from build123d import *

# Parameters (mm, degrees)
F0_W      = 80
F0_H      = 70
F1_DEPTH  = 2
F2_W      = 80
F2_H      = 140
F3_DEPTH  = 2
F4_W      = 140
F4_H      = 68
F5_DEPTH  = 2
F6_W      = 140
F6_H      = 68
F7_DEPTH  = 2
F8_R      = 2
F9_DEPTH  = 2
F10_R     = 2
F11_R     = 1.5
F12_DEPTH = 4
F13_DEPTH = 8
F14_DEPTH = 8
F15_W     = 2
F15_H     = 68
F16_DEPTH = 3
F17_W     = 2
F17_H     = 68
F18_DEPTH = 3


with BuildPart() as f1:
    # F0 (on Front) → F1 (new body)
    with BuildSketch(Plane.XZ):
        with Locations((0, 35)):
            Rectangle(F0_W, F0_H)
    extrude(amount=F1_DEPTH)

    # F2 (on Top) → F3 (join)
    with BuildSketch(Plane.XY):
        with Locations((0, 70)):
            Rectangle(F2_W, F2_H)
    extrude(amount=F3_DEPTH)

    # F4 (on face) → F5 (join)
    with BuildSketch(Plane(origin=(-40, 0, 0), x_dir=(0, -1, 0), z_dir=(-1, 0, 0))):
        with Locations((-70, 36)):
            Rectangle(F4_W, F4_H)
    extrude(amount=-F5_DEPTH)

    # F6 (on face) → F7 (join)
    with BuildSketch(Plane.YZ.offset(40)):
        with Locations((70, 36)):
            Rectangle(F6_W, F6_H)
    extrude(amount=-F7_DEPTH)

    # F8 (on face) → F9 (cut)
    with BuildSketch(Plane.XZ.offset(2)):
        with BuildLine():
            Line((-9.5176118745, 43.1033983122), (-15.8934493297, 49.4792357673))
            ThreePointArc((-15.8934493297, 49.4792357673), (-21.4980117445, 34.7076115032), (-15.4937871876, 20.0938751318))
            Line((-15.4937871876, 20.0938751318), (-9.2937080159, 26.640754142))
            ThreePointArc((-9.2937080159, 26.640754142), (-12.4988440375, 34.8300066879), (-9.5176118745, 43.1033983122))
        make_face()
        with BuildLine():
            Line((-16.6012881064, 50.1870745441), (-21.2010083131, 54.7867947507))
            ThreePointArc((-21.2010083131, 54.7867947507), (-28.997318167, 34.6056155159), (-20.6550363783, 14.6439327912))
            Line((-20.6550363783, 14.6439327912), (-16.1821134643, 19.3670475013))
            ThreePointArc((-16.1821134643, 19.3670475013), (-22.4979192675, 34.6940120382), (-16.6012881064, 50.1870745441))
        make_face()
        with Locations((-26, 61)):
            Circle(F8_R)
        with BuildLine():
            ThreePointArc((19.2028843822, 56.731296128), (-0.3943844841, 63.997318167), (-19.7867947507, 56.2010083131))
            Line((-19.7867947507, 56.2010083131), (-15.1870745441, 51.6012881064))
            ThreePointArc((-15.1870745441, 51.6012881064), (-0.3059879618, 57.4979192675), (14.7299614682, 52.0081814179))
            Line((14.7299614682, 52.0081814179), (19.2028843822, 56.731296128))
        make_face()
        with BuildLine():
            ThreePointArc((14.0416351915, 51.2813537874), (-0.2923884968, 56.4980117445), (-14.4792357673, 50.8934493297))
            Line((-14.4792357673, 50.8934493297), (-8.1033983122, 44.5176118745))
            ThreePointArc((-8.1033983122, 44.5176118745), (-0.1699933121, 47.4988440375), (7.8415560198, 44.7344747772))
            Line((7.8415560198, 44.7344747772), (14.0416351915, 51.2813537874))
        make_face()
        with BuildLine():
            Line((9.5176118745, 26.8966016878), (15.8934493297, 20.5207642327))
            ThreePointArc((15.8934493297, 20.5207642327), (21.5, 35), (15.8934493297, 49.4792357673))
            Line((15.8934493297, 49.4792357673), (9.5176118745, 43.1033983122))
            ThreePointArc((9.5176118745, 43.1033983122), (12.5, 35), (9.5176118745, 26.8966016878))
        make_face()
        with BuildLine():
            Line((21.2010083131, 54.7867947507), (16.6012881064, 50.1870745441))
            ThreePointArc((16.6012881064, 50.1870745441), (22.5, 35), (16.6012881064, 19.8129254559))
            Line((16.6012881064, 19.8129254559), (21.2010083131, 15.2132052493))
            ThreePointArc((21.2010083131, 15.2132052493), (29, 35), (21.2010083131, 54.7867947507))
        make_face()
        with Locations((26, 61)):
            Circle(F8_R)
        with Locations((26, 9)):
            Circle(F8_R)
        with BuildLine():
            Line((-15.1870745441, 18.3987118936), (-19.7867947507, 13.7989916869))
            ThreePointArc((-19.7867947507, 13.7989916869), (0, 6), (19.7867947507, 13.7989916869))
            Line((19.7867947507, 13.7989916869), (15.1870745441, 18.3987118936))
            ThreePointArc((15.1870745441, 18.3987118936), (0, 12.5), (-15.1870745441, 18.3987118936))
        make_face()
        with BuildLine():
            ThreePointArc((8.1033983122, 25.4823881255), (0, 22.5), (-8.1033983122, 25.4823881255))
            Line((-8.1033983122, 25.4823881255), (-14.4792357673, 19.1065506703))
            ThreePointArc((-14.4792357673, 19.1065506703), (0, 13.5), (14.4792357673, 19.1065506703))
            Line((14.4792357673, 19.1065506703), (8.1033983122, 25.4823881255))
        make_face()
        with Locations((-26, 9)):
            Circle(F8_R)
    extrude(amount=-F9_DEPTH, mode=Mode.SUBTRACT)

    # F10
    f10_edges = [f1.edges().sort_by_distance(p)[0] for p in [
        (40, 69, 0),
        (-40, 69, 0),
    ]]
    fillet(f10_edges, radius=F10_R)

    # F11 (on face) → F12 (join)
    with BuildSketch(Plane.XY.offset(2)):
        with BuildLine():
            ThreePointArc((-21.15, 117.6), (-23.2839745962, 120.4722813233), (-26.65, 119.2583123952))
            Line((-26.65, 119.2583123952), (-26.65, 115.9416876048))
            ThreePointArc((-26.65, 115.9416876048), (-23.2839745962, 114.7277186767), (-21.15, 117.6))
        make_face()
        with Locations((-24.15, 117.6)):
            Circle(F11_R, mode=Mode.SUBTRACT)
        with BuildLine():
            Line((26.65, 114.6416876048), (26.65, 117.9583123952))
            ThreePointArc((26.65, 117.9583123952), (21.15, 116.3), (26.65, 114.6416876048))
        make_face()
        with Locations((24.15, 116.3)):
            Circle(F11_R, mode=Mode.SUBTRACT)
        with BuildLine():
            ThreePointArc((-21.15, 35), (-23.2839745962, 37.8722813233), (-26.65, 36.6583123952))
            Line((-26.65, 36.6583123952), (-26.65, 33.3416876048))
            ThreePointArc((-26.65, 33.3416876048), (-23.2839745962, 32.1277186767), (-21.15, 35))
        make_face()
        with Locations((-24.15, 35)):
            Circle(F11_R, mode=Mode.SUBTRACT)
        with BuildLine():
            Line((26.65, 39.7416876048), (26.65, 43.0583123952))
            ThreePointArc((26.65, 43.0583123952), (21.15, 41.4), (26.65, 39.7416876048))
        make_face()
        with Locations((24.15, 41.4)):
            Circle(F11_R, mode=Mode.SUBTRACT)
        with Locations((24.15, 116.3)):
            Circle(F11_R)
        with BuildLine():
            ThreePointArc((27.15, 116.3), (27.0222813233, 117.1660254038), (26.65, 117.9583123952))
            Line((26.65, 117.9583123952), (26.65, 114.6416876048))
            ThreePointArc((26.65, 114.6416876048), (27.0222813233, 115.4339745962), (27.15, 116.3))
        make_face()
        with BuildLine():
            Line((-26.65, 115.9416876048), (-26.65, 119.2583123952))
            ThreePointArc((-26.65, 119.2583123952), (-27.15, 117.6), (-26.65, 115.9416876048))
        make_face()
        with BuildLine():
            ThreePointArc((27.15, 41.4), (27.0222813233, 42.2660254038), (26.65, 43.0583123952))
            Line((26.65, 43.0583123952), (26.65, 39.7416876048))
            ThreePointArc((26.65, 39.7416876048), (27.0222813233, 40.5339745962), (27.15, 41.4))
        make_face()
        with BuildLine():
            Line((-26.65, 33.3416876048), (-26.65, 36.6583123952))
            ThreePointArc((-26.65, 36.6583123952), (-27.15, 35), (-26.65, 33.3416876048))
        make_face()
    extrude(amount=F12_DEPTH)

    # F11 (on face) → F13 (join)
    with BuildSketch(Plane.XY.offset(2)):
        with Locations((-24.15, 35)):
            Circle(F11_R)
        with Locations((-24.15, 117.6)):
            Circle(F11_R)
    extrude(amount=F13_DEPTH)

    # F11 (on face) → F14 (join)
    with BuildSketch(Plane.XY.offset(2)):
        with Locations((24.15, 41.4)):
            Circle(F11_R)
    extrude(amount=F14_DEPTH)

    # F15 (on face) → F16 (join)
    with BuildSketch(Plane(origin=(38, 0, 0), x_dir=(0, -1, 0), z_dir=(-1, 0, 0))):
        with Locations((-117, 36)):
            Rectangle(F15_W, F15_H)
        with Locations((-21, 36)):
            Rectangle(F15_W, F15_H)
    extrude(amount=F16_DEPTH)

    # F17 (on face) → F18 (join)
    with BuildSketch(Plane.YZ.offset(-38)):
        with Locations((21, 36)):
            Rectangle(F17_W, F17_H)
        with Locations((117, 36)):
            Rectangle(F17_W, F17_H)
    extrude(amount=F18_DEPTH)


solid = f1.part
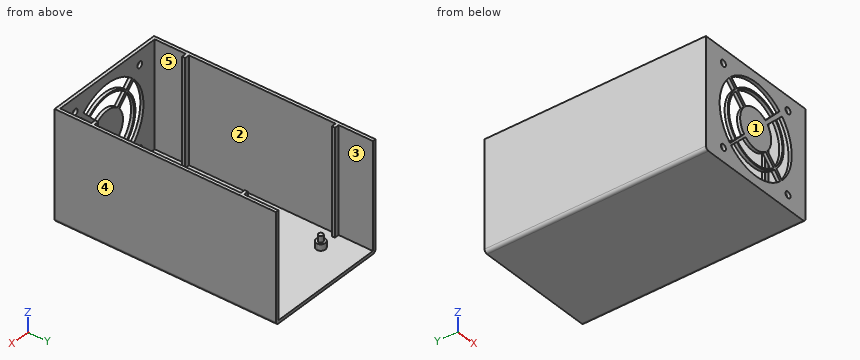
Geometry: final body of the model. Coordinates: model frame, mm. Face numbers are marked on the shaded views. A direction names the side the tool comes from. Give positions to 0.01 mm unless a question says otherwise; leave off trailing zeros. Write each loop counter-clockwise with the first axis right and the second up, starting at its lowest first coordinate (ties: lowest second). Pieces come first, ordered by that corner, then holes. Notation, with made-up numbers: (14, -8.75) - (18, -8.75) arc R18 ccw to (18, 0.25) - close; hole circle Ø8 at (-16, 3.5). An arc over 180 degrees is marked (long way). Return JSON: item names as keys, results as strings. Group by question number.
1) Line query: line 1 (X direction, y = 57.5, z = 31); line 2 (Z direction, x = -26, y = -1.25); line 3 (Y direction, x = 23, z = 17). Output: solid intervals per line, ascending.
2) Mould query, pull axis Y, two halves, no side actions, for the marked faces 1, 2 and 3. Classes: released by +Y, released by -Y, zero draft, split by the parting line, or undercut.
3) Set-up query: the marked faces 4 and 5. Return all of +Z, -Z, +X, -X, +Y, -Y with unobstructed straight access to the full face (end or side cutting, diameter ignored); none if empty.
4) Section A-A on x = -2. Return the cut outline in (y, z).
5) Section B-B on y = 17. Return the cut outline in (x, z), plus the area to 3 significant figures.
6) First-contact query: P1, Ø4.5, axis at x = -26, z = 61, coming from the +Y side; P2, Ø2.5, axis at x = -37, z = 48.5, coming from the +Y side; P3, Ø2, axis at x = -11, y = 64.5, coming from the +Z side; P4, Ø0.9, axis at x = -24, y = 35.5, coming from the +Z side. Flat tips, straight axial feed; report the tip coordinate or a pass-through.
7) Section C-C on z = 61. State how many separate pieces and enclosed holes the cut face has, plus the area to 3 significant figures.
Filled in:
{
 "1": {"line 1": "x = -40 to -38, 38 to 40", "line 2": "z = 0 to 7, 11 to 22.15, 47.85 to 59, 63 to 70", "line 3": "y = -2 to 0"},
 "2": {"face 1": "released by -Y", "face 2": "undercut", "face 3": "zero draft"},
 "3": {"face 4": "+Z, -Z, +X, +Y, -Y", "face 5": "+Z"},
 "4": {"outline": "(-2, 0) - (140, 0) - (140, 2) - (0, 2) - (0, 6.07) - (-2, 6.07) - close; (-2, 12.59) - (0, 12.59) - (0, 13.59) - (-2, 13.59) - close; (-2, 22.66) - (0, 22.66) - (0, 47.34) - (-2, 47.34) - close; (-2, 56.41) - (0, 56.41) - (0, 57.41) - (-2, 57.41) - close; (-2, 63.93) - (0, 63.93) - (0, 70) - (-2, 70) - close"},
 "5": {"outline": "(-40, 2) arc R2 ccw to (-38, 0) - (38, 0) arc R2 ccw to (40, 2) - (40, 70) - (38, 70) - (38, 2) - (-38, 2) - (-38, 70) - (-40, 70) - close", "area": "430 mm^2"},
 "6": {"P1": "stops at y = 0", "P2": "stops at y = 140", "P3": "stops at z = 2", "P4": "stops at z = 10"},
 "7": {"separate pieces": "4", "enclosed holes": "0", "area": "677 mm^2"}
}
